from build123d import *
from OCP.BRepFilletAPI import BRepFilletAPI_MakeChamfer

# Parameters (mm, degrees)
BOSS_EXTRUDE1_DEPTH         = 35.56
SKETCH2_W                   = 12.59949555
SKETCH2_H                   = 5.842
CUT_EXTRUDE1_DEPTH          = 12.7
CUT_EXTRUDE2_DEPTH          = 12.7
F_1_4_20_TAPPED_HOLE1_D     = 5.1054
F_1_4_20_TAPPED_HOLE1_DEPTH = 14.086183098
F_1_4_20_TAPPED_HOLE1_TIP   = 1.533816902
CHAMFER1_SIZE               = 1.2192
CHAMFER1_SIZE2              = 3.330916345


with BuildPart() as part:
    # Sketch1 → Boss-Extrude1 (new body)
    with BuildSketch(Plane(origin=(0, 0, 0), x_dir=(1, 0, 0), z_dir=(0, 1, 0))):
        Polygon((-14.664696837, 0), (-7.332348419, -12.7), (7.332348419, -12.7), (14.664696837, 0), (7.332348419, 12.7), (-7.332348419, 12.7), align=None)
    extrude(amount=BOSS_EXTRUDE1_DEPTH)

    # Sketch2 → Cut-Extrude1 (cut)
    with BuildSketch(Plane(origin=(0, 35.56, 0), x_dir=(1, 0, 0), z_dir=(0, 1, 0))):
        Rectangle(SKETCH2_W, SKETCH2_H)
    extrude(amount=-CUT_EXTRUDE1_DEPTH, mode=Mode.SUBTRACT)

    # Sketch3 → Cut-Extrude2 (cut)
    with BuildSketch(Plane.XZ):
        Polygon((0, 6.465784407), (-6.465784407, 0), (0, -6.465784407), (6.465784407, 0), align=None)
    extrude(amount=-CUT_EXTRUDE2_DEPTH, mode=Mode.SUBTRACT)

    # 1/4-20 Tapped Hole1
    with Locations(Plane.XY.offset(12.7)):
        with Locations((0, 29.21)):
            Hole(F_1_4_20_TAPPED_HOLE1_D / 2, depth=F_1_4_20_TAPPED_HOLE1_DEPTH)
            with Locations((0, 0, -(F_1_4_20_TAPPED_HOLE1_DEPTH + F_1_4_20_TAPPED_HOLE1_TIP / 2))):  # 118° drill point
                Cone(0, F_1_4_20_TAPPED_HOLE1_D / 2, F_1_4_20_TAPPED_HOLE1_TIP, mode=Mode.SUBTRACT)

    # Chamfer1: one chamfer whose edges measure the first distance from different faces: ONE call of the kernel's chamfer builder (chamfer() names one face for all edges)
    chamfer1_edges_1 = [part.edges().sort_by_distance(p)[0] for p in [
        (-7.332348419, 17.78, -12.7),
    ]]
    chamfer1_side_1 = [part.faces().sort_by_distance(p)[0] for p in [
        (0, 17.78, -12.7),
    ]]
    chamfer1_edges_2 = [part.edges().sort_by_distance(p)[0] for p in [
        (7.332348419, 17.78, -12.7),
    ]]
    chamfer1_side_2 = [part.faces().sort_by_distance(p)[0] for p in [
        (10.998522628, 17.78, -6.35),
    ]]
    chamfer1_edges_3 = [part.edges().sort_by_distance(p)[0] for p in [
        (14.664696837, 17.78, 0),
    ]]
    chamfer1_side_3 = [part.faces().sort_by_distance(p)[0] for p in [
        (10.998522628, 17.78, 6.35),
    ]]
    chamfer1_edges_4 = [part.edges().sort_by_distance(p)[0] for p in [
        (7.332348419, 17.78, 12.7),
    ]]
    chamfer1_side_4 = [part.faces().sort_by_distance(p)[0] for p in [
        (0, 17.312960636, 12.7),
    ]]
    chamfer1_edges_5 = [part.edges().sort_by_distance(p)[0] for p in [
        (-7.332348419, 17.78, 12.7),
    ]]
    chamfer1_side_5 = [part.faces().sort_by_distance(p)[0] for p in [
        (-10.998522628, 17.78, 6.35),
    ]]
    chamfer1_edges_6 = [part.edges().sort_by_distance(p)[0] for p in [
        (-14.664696837, 17.78, 0),
    ]]
    chamfer1_side_6 = [part.faces().sort_by_distance(p)[0] for p in [
        (-10.998522628, 17.78, -6.35),
    ]]
    chamfer1_edges_7 = [part.edges().sort_by_distance(p)[0] for p in [
        (0, 6.35, -6.465784407),
        (-6.465784407, 6.35, 0),
        (0, 6.35, 6.465784407),
        (6.465784407, 6.35, 0),
    ]]
    chamfer1 = BRepFilletAPI_MakeChamfer(part.part.solid().wrapped)
    for e in chamfer1_edges_1:
        chamfer1.Add(CHAMFER1_SIZE, CHAMFER1_SIZE2, e.wrapped, chamfer1_side_1[0].wrapped)  # the first distance lies on this face
    for e in chamfer1_edges_2:
        chamfer1.Add(CHAMFER1_SIZE, CHAMFER1_SIZE2, e.wrapped, chamfer1_side_2[0].wrapped)  # the first distance lies on this face
    for e in chamfer1_edges_3:
        chamfer1.Add(CHAMFER1_SIZE, CHAMFER1_SIZE2, e.wrapped, chamfer1_side_3[0].wrapped)  # the first distance lies on this face
    for e in chamfer1_edges_4:
        chamfer1.Add(CHAMFER1_SIZE, CHAMFER1_SIZE2, e.wrapped, chamfer1_side_4[0].wrapped)  # the first distance lies on this face
    for e in chamfer1_edges_5:
        chamfer1.Add(CHAMFER1_SIZE, CHAMFER1_SIZE2, e.wrapped, chamfer1_side_5[0].wrapped)  # the first distance lies on this face
    for e in chamfer1_edges_6:
        chamfer1.Add(CHAMFER1_SIZE, CHAMFER1_SIZE2, e.wrapped, chamfer1_side_6[0].wrapped)  # the first distance lies on this face
    for e in chamfer1_edges_7:
        chamfer1.Add(CHAMFER1_SIZE, e.wrapped)
    add(Compound.cast(chamfer1.Shape()), mode=Mode.REPLACE)


solid = part.part
The listing builds one solid part. Answer for the finished solid, in the listing's coordinates (mm). A direction names the side the tool comes from. Give positions to 0.01 mm unless a question says otherwise; leave off trailing zeros. Write each loop counter-clockwise with the first axis right and the second up, starting at its lowest first coordinate (ties: lowest second). Pieces come first, ordered by that corner, then holes. Notation, with made-up numbers: (-5, -35) - (25, -35) arc R30 cw to (25, -12) - close; hole circle Ø6 at (21, 37). An arc over 180 degrees is marked (long way). Use a Markdown table: item, result.
1. A tool of negligible diameter and unlimited length cuts with its end or side. For faces 4 (the flat face through (-6.3, 29, 0)), 5 (the cylindrical face through (-1.372, 31.362, 7.742)), 6 (the flat face through (3.266, 6.261, 3.2)), from which of +Z, -Z, +X, -X, +Y, -Y can it reach the whole face along a straight path? Write none if from no direction.
Values follow:
| item | result |
|---|---|
| face 4 | +Y |
| face 5 | +Z |
| face 6 | -Y |
2. Section D-D on z = -4.25 is taken. Write down the section's boundary in (x, y).
Values follow:
| item | result |
|---|---|
| outline | (-12.21, 0) - (-2.22, 0) - (-2.22, 12.7) - (2.22, 12.7) - (2.22, 0) - (12.21, 0) - (12.21, 35.56) - (-12.21, 35.56) - close |
3. Each of these flat-tipped pins is pushed along its axis until it touches: P1, Ø1.4, axis at y = 7, z = -0.5, coming from the +X side; P2, Ø4, axis at y = 4.5, z = -6.5, coming from the -X side; P3, Ø3, axis at y = 26.5, z = -0.5, coming from the +X side. Where does it stop, or does it pass through?
Values follow:
| item | result |
|---|---|
| P1 | stops at x = 13.83 |
| P2 | stops at x = -12.07 |
| P3 | stops at x = 14.04 |
4. Section C-C on z = 8 is taken. Write down the section's boundary in (x, y), plus the area to 3 significant figures.
Values follow:
| item | result |
|---|---|
| outline | (-10.05, 0) - (10.05, 0) - (10.05, 35.56) - (-10.05, 35.56) - close; hole circle Ø5.11 at (0, 29.21) |
| area | 694 mm² |
5. Section A-A on x = 0 is taken. Write down the section's boundary in (y, z).
Values follow:
| item | result |
|---|---|
| outline | (0, -12.7) - (35.56, -12.7) - (35.56, -2.92) - (22.86, -2.92) - (22.86, 2.92) - (26.66, 2.92) - (26.66, 12.7) - (0, 12.7) - (0, 5.6) - (12.7, 5.6) - (12.7, -5.6) - (0, -5.6) - close; (31.76, 2.92) - (35.56, 2.92) - (35.56, 12.7) - (31.76, 12.7) - close |
6. For a pull along X with two mould halves and no side action, classify faces 1 (the flat face through (0, 35.56, -6)), 2 (the flat face through (0, 12.7, 0)), 3 (the flat face through (10.51, 17.53, -7.2)) as released by +X, released by -X, zero draft, split by the parting line, or undercut.
Values follow:
| item | result |
|---|---|
| face 1 | zero draft |
| face 2 | undercut |
| face 3 | released by +X |
7. Find the intervals of material crossed by probe 1 along Y at (x, z) = (0, 10.75); probe 2 along Z at (x, y) = (3.5, 23); probe 3 along Z at (x, y) = (-0.75, 4), in increasing order. Write a range as from..to.
Values follow:
| item | result |
|---|---|
| probe 1 | y = 0..26.66, 31.76..35.56 |
| probe 2 | z = -12.7..-2.92, 2.92..12.7 |
| probe 3 | z = -12.7..-5.6, 5.6..12.7 |
8. Section B-B on y = 14 is taken. Write down the section's boundary in (x, z).
Values follow:
| item | result |
|---|---|
| outline | (-14.06, -1.06) - (-9, -9.82) - (-6.11, -12.7) - (4, -12.7) - (7.94, -11.64) - (13, -2.88) - (14.06, 1.06) - (9, 9.82) - (6.11, 12.7) - (-4, 12.7) - (-7.94, 11.64) - (-13, 2.88) - close |
